Autodesk Inventor part; units mm, degrees
ref_plane "YZ Plane" through (0, 0, 0) normal (1, 0, 0) x (0, 1, 0)
ref_plane "XZ Plane" through (0, 0, 0) normal (0, 1, 0) x (-1, 0, 0)
ref_plane "XY Plane" through (0, 0, 0) normal (0, 0, 1) x (1, 0, 0)
sketch "Sketch2" plane through (0, 0, 0) normal (0, 1, 0) x (-1, 0, 0)
  circle A0 centre (0, 0) radius 2.5
  circle A1 centre (0, 0) radius 1.4
  dimension "d9" = 5
  dimension "d10" = 2.8
sketch "Sketch1" plane through (0, 0, 0) normal (0, 0, 1) x (1, 0, 0)
  line L0 (-1.7856, -0.1072) -> (0.9856, 1.4928)
  line L1 (0.9856, 1.4928) -> (1.7856, 0.1072)
  line L2 (1.7856, 0.1072) -> (-0.9856, -1.4928)
  line L3 (-0.9856, -1.4928) -> (-1.7856, -0.1072)
  line L4 (0.9856, 1.4928) -> (-0.9856, -1.4928) construction
  line L5 (0, -2.0899) -> (0, 2.0899) construction
  line L6 (-2.4999, 0) -> (2.4999, 0) construction
  point P0 (0, 0)
  dimension "d0" = 1.6
  dimension "d1" = 3.2
  dimension "d2" = 30
extrude "Extrusion1" add sketch "Sketch1" along normal blind 15
fillet "Fillet1" radius 1.6 2 edges at (1.3856, 0.8, 15) (-1.3856, -0.8, 15)
pattern_circular "Circular Pattern1" count 3 over 360 about axis through (0, -10, 0) along (0, 1, 0) of "Extrusion1", "Fillet1"
extrude "Extrusion2" add sketch "Sketch2" along normal mid plane 3.2 contours A0 | A1
extrude "Extrusion3" cut sketch "Sketch2" along normal through all both and the other way through all contours A1
equation "\"d5\" = 0.5 * d1"
properties part number "LEGO Brick 2421" material "Steel"
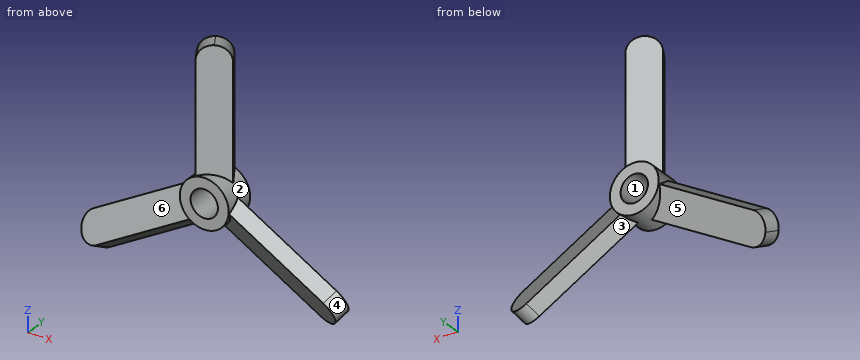
Verification items for the finished model (mm, model axes). Face numbers are marked on the shaded views. A direction names the side the tool comes from. Round coordinates to 2 decimals unless told otherwise and drop trailing zeros. Write each loop counter-clockwise with the first axis right and the second up, starting at its lowest first coordinate (ties: lowest second). Pieces come first, ordered by that corner, then holes.
1. Gauge pin test, flat end, axial feed: P1, Ø1.7, axis at x = 0, z = 0, coming from the +Y side. Record the tip position at first contact, or that the pin passes through.
2. Draft check along X on the marked faces 4, 5 and 6. Enter one of: +X half, -X half, draft (parallel to the pull), parting line (faces both ways), or undercut.
3. Section check A-A on z = 0. Enter the section's corners in (x, y).
4. Access from +Z, -Z, +X, -X, +Y, -Y to the whole of each face (thin tool, end or side, straight path). Record for the marked faces 1, 2 and 3.
5. Section check C-C on x = -4. Enter the section's corners in (y, z), plus the area to 3 significant figures.
6. Scan lines: L1, parallel to X at y = 0.65, z = 0; L2, parallel to X at y = 0.55, z = 0; L3, parallel to X at y = 1.25, z = 3. Record each from-to range of solid material in increasing order.
7. Section check B-B on z = 6. Enter the section's corners in (x, y), plus the area to 3 significant figures.
Answer:
1. P1: passes through
2. face 4: +X half
2. face 5: undercut
2. face 6: -X half
3. outline: (-3.57, 0.11) - (-2.5, -0.2) - (-2.5, -1.6) - (-1.4, -1.6) - (-1.4, 1.6) - (-2.5, 1.6) - (-2.5, 1.03) - close; (1.4, -1.6) - (2.5, -1.6) - (2.5, -1.03) - (3.57, -0.11) - (2.5, 0.2) - (2.5, 1.6) - (1.4, 1.6) - close
4. face 1: +Y, -Y
4. face 2: none
4. face 3: -Z, +Y
5. outline: (-1.49, -3.45) - (-0.11, -4.37) - (1.49, -1.17) - (0.11, -0.25) - close
5. area: 5.91 mm2
6. L1: x = -2.94 to -1.4, 1.4 to 2.5
6. L2: x = -3.06 to -1.4, 1.4 to 2.5
6. L3: x = 0.57 to 1.13
7. outline: (-1.79, -0.11) - (-0.99, -1.49) - (1.79, 0.11) - (0.99, 1.49) - close
7. area: 5.12 mm2
